Geometry check sheet. Reference: the model listing, model coordinates, mm. A direction names the side the tool comes from. Coordinates: 2 decimals unless noted, no trailing zeros. Loops run counter-clockwise (first coordinate to the right, second up) from the corner with the lowest first, then second, coordinate; pieces in that order, holes last.
from build123d import *

# Parameters (mm, degrees)
CUT_EXTRUDE1_DEPTH      = 90.050468029
CUT_EXTRUDE1_DEPTH_BACK = 90.050468029
SKETCH3_W               = 27.181091561
SKETCH3_H               = 38.454465552


# Read off the part's stored shape, not the designer's step: Shell2
with BuildPart() as part:
    # Sketch1 → Revolve1 (revolve)
    with BuildSketch(Plane.XY, mode=Mode.PRIVATE) as revolve1_sk:
        with BuildLine():
            Line((0, 0), (0, -50.8))
            ThreePointArc((0, -50.8), (3.280951188, -68.760512242), (12.7, -84.401041651))
            Line((12.7, -84.401041651), (12.7, 0))
            Line((12.7, 0), (0, 0))
        make_face()
    revolve(revolve1_sk.sketch.rotate(Axis((12.7, -84.401041651, 0), (0, 1, 0)), 180), axis=Axis((12.7, -84.401041651, 0), (0, 1, 0)))

    # Shell2 outline → Shell2 (revolve, cut)
    with BuildSketch(Plane(origin=(12.7, 0, 0), x_dir=(1, 0, 0), z_dir=(0, 0, 1))):
        with BuildLine():
            Line((0, 0), (0, -76.642627696))
            add(Edge.make_bspline(
                [(7.9375, -50.8), (7.9375, -64.940305721), (0, -76.642627696)],
                knots=[0, 0, 0, 0.596002439, 0.596002439, 0.596002439], degree=2, weights=[1, 0.95592526, 1]))
            Line((7.9375, -50.8), (7.9375, 0))
            Line((7.9375, 0), (0, 0))
        make_face()
    revolve(axis=Axis((12.7, 0, 0), (0, 1, 0)), mode=Mode.SUBTRACT)

    # Sketch3 → Cut-Extrude1 (cut, two sides: drawn at the far end of the back side and taken through both)
    with BuildSketch(Plane.XY.offset(-CUT_EXTRUDE1_DEPTH_BACK)):
        with Locations((13.590545781, -70.027232776)):
            Rectangle(SKETCH3_W, SKETCH3_H)
    extrude(amount=CUT_EXTRUDE1_DEPTH + CUT_EXTRUDE1_DEPTH_BACK, mode=Mode.SUBTRACT)

    # Sketch2 → Revolve3 (revolve)
    with BuildSketch(Plane.XY, mode=Mode.PRIVATE) as revolve3_sk:
        with BuildLine():
            Line((12.7, -82.559521115), (12.7, -50.8))
            Line((12.7, -50.8), (0, -50.8))
            ThreePointArc((0, -50.8), (1.730968025, -63.948007491), (6.805909488, -76.2))
            Line((6.805909488, -76.2), (10.047183612, -81.128995309))
            ThreePointArc((10.047183612, -81.128995309), (11.193029623, -82.179098952), (12.7, -82.559521115))
        make_face()
    revolve(revolve3_sk.sketch.rotate(Axis((12.7, -82.559521115, 0), (0, 1, 0)), 180), axis=Axis((12.7, -82.559521115, 0), (0, 1, 0)))


solid = part.part
1) Depth check by flat-ended pin: pin 1 (12 mm diameter, centred on x = 11, z = 6.5, fed in from +Y); pin 2 (1.5 mm diameter, centred on x = 19.5, y = -12.5, fed in from +Z); pin 3 (8 mm diameter, centred on x = 4, z = 6.5, fed in from -Y); pin 4 (6 mm diameter, centred on y = -54, z = 3.5, fed in from +X). Enter the tip coordinate at first touch or a pass-through.
Data:
pin 1: stops at y = 0
pin 2: stops at z = 11.17
pin 3: stops at y = -74.45
pin 4: stops at x = 25.34
2) Section check A-A on y = -30.5. Record the cut outline in (x, z) (1 decimal), and give its area (3 significant figures).
Data:
outline: circle Ø25.4 at (12.7, 0); hole circle Ø15.9 at (12.7, 0)
area: 309 mm2
3) Material ranges on probe 1 along Z at (x, y) = (12.7, -17); probe 2 along X at (y, z) = (-44, 7); probe 3 along X at (y, z) = (-25, 4.5), recorded low to high.
Data:
probe 1: z = -12.7 to -7.94, 7.94 to 12.7
probe 2: x = 2.1 to 8.96, 16.44 to 23.3
probe 3: x = 0.82 to 6.16, 19.24 to 24.58
4) Mould release check, pull along X, two halves, no side actions. Record for faces 3 (the cylindrical face through (20.271, -25.044, -2.384)), 4 (the flat face through (7, 0, -6)), 5 (the conical face through (15.296, -80.89, 1.076)): +X half, -X half, draft (parallel to the pull), parting line (faces both ways), or undercut.
Data:
face 3: undercut
face 4: draft
face 5: parting line
5) Access from +Z, -Z, +X, -X, +Y, -Y to the whole of each face (thin tool, end or side, straight path). Record for faces 1 (the cylindrical face through (18.56, -25.756, 11.267)), 2 (the flat face through (13, -50.8, 0)).
Data:
face 1: +Y, -Y
face 2: +Y
